For this review, take the finished solid that the model builds, in its own axes (mm). A direction names the side the tool comes from. Give positions to 0.01 mm unless a question says otherwise; leave off trailing zeros. Order: outer loops, then holes, each group sorted by start corner. A loop starts at its lowest first (then second) coordinate and runs counter-clockwise, first axis right, second up. Notation, with made-up numbers: (50, -39.5) -> (72, -39.5) arc R34 ccw to (72, -7.5) -> close; hole circle Ø5 at (20.25, 22.25). An arc over 180 degrees is marked (long way). Return JSON: item names as keys, results as strings. Group by question number.
1) Insertion check: P1, Ø2, axis at y = -1, z = 20.5, coming from the -X side; P2, Ø12.5, axis at x = 149.5, y = 38, coming from the -Z side; P3, Ø1, axis at y = -1, z = -153.5, coming from the +X side. Each pin has a flat end and moves straight along its axis. Give the tip position at first contact, or say it passes through.
2) The part is to be moulded in two halves that separate along Z. For faces 1 (the face through (159, 0, -2)), 2 (the face through (156.7, -1, 159.9)), say which applies: released by +Z, released by -Z, zero draft, split by the parting line, or undercut.
3) Add section C-C (z = 35.5). Give the boundary of the cut face in (x, y).
4) For faces 3 (the face through (159, -2, -2)), 4 (the face through (155.116, 34.439, 1.568)), list the 3-axis set-ups (+Z, -Z, +X, -X, +Y, -Y) from which the entire face can be reached by the end or side of a thin tool; tool diameter is ignored.
5) To check wall thickness, follow line 1 along Z through (x, y) = (160, -0.85); line 2 along X through (y, z) = (-1.5, -160); line 3 along Y through (x, z) = (147, 70). State the ranges of each line that lie inside material, in increasing order.
6) Add section B-B (x = 167). Give the boundary of the cut face in (y, z).
7) Add section A-A (z = 160). Give the boundary of the cut face in (x, y), then the cut area to 3 significant figures.
8) Add section D-D (z = 126). Give the boundary of the cut face in (x, y).
from build123d import *

# Parameters (mm, degrees)
SKIZZE2_W                       = 350
SKIZZE2_H                       = 335
BASIS_BLECH1_DEPTH              = 2
KANTE_LASCHE1_STRIP_CUT_DEPTH   = 224
KANTE_LASCHE1_RELIEF_W          = 14.502816622
KANTE_LASCHE1_RELIEF_H          = 0.3
KANTE_LASCHE1_RELIEF_CUT_DEPTH  = 2
KANTE_LASCHE1_DEPTH             = 224
DURCHGANGSLOCH_F_R_M61_D        = 6.6
DURCHGANGSLOCH_F_R_M61_DEPTH    = 15
DURCHGANGSLOCH_F_R_M61_TIP      = 1.982840043
DURCHGANGSLOCH_F_R_M121_D       = 13.5
SKIZZE30_W                      = 319
SKIZZE30_H                      = 335
SCHNITT_LINEAR_AUSTRAGEN1_DEPTH = 10


# Sheet-metal steps are written as plain solids
with BuildPart() as part:
    # Skizze2 → Basis-Blech1 (new body)
    with BuildSketch(Plane(origin=(0, 0, 0), x_dir=(1, 0, 0), z_dir=(0, 1, 0))):
        Rectangle(SKIZZE2_W, SKIZZE2_H)
    extrude(amount=-BASIS_BLECH1_DEPTH)

    # Kante-Lasche1 strip (across the edge) → Kante-Lasche1 strip cut (cut)
    with BuildSketch(Plane(origin=(175, 0, 112), x_dir=(-0.8660254037844407, -0.49999999999999645, 0), z_dir=(0, 0, -1))):
        Polygon((-11.15, -8.746856578), (1.15, -1.645448267), (0.15, 0.08660254), (-12.15, -7.014805771), align=None)
    extrude(amount=KANTE_LASCHE1_STRIP_CUT_DEPTH, mode=Mode.SUBTRACT)

    # Kante-Lasche1 relief (on the sheet) → Kante-Lasche1 relief cut (cut)
    with BuildSketch(Plane(origin=(174.826794919, 0, 112), x_dir=(-1, 0, 0), z_dir=(0, 1, 0))):
        with Locations((-6.951408311, 0.15)):
            Rectangle(KANTE_LASCHE1_RELIEF_W, KANTE_LASCHE1_RELIEF_H)
        with Locations((-6.951408311, -224.15)):
            Rectangle(KANTE_LASCHE1_RELIEF_W, KANTE_LASCHE1_RELIEF_H)
    extrude(amount=-KANTE_LASCHE1_RELIEF_CUT_DEPTH, mode=Mode.SUBTRACT)

    # Kante-Lasche1 section (across the edge) → Kante-Lasche1 (add)
    with BuildSketch(Plane(origin=(175, 0, 112), x_dir=(-0.8660254037844407, -0.49999999999999645, 0), z_dir=(0, 0, -1))):
        with BuildLine():
            Line((-2, 0.173205081), (-2, 78.267949192))
            Line((-2, 78.267949192), (0, 78.267949192))
            Line((0, 78.267949192), (0, 0.173205081))
            ThreePointArc((0, 0.173205081), (0.05, 0.08660254), (0.15, 0.08660254))
            Line((0.15, 0.08660254), (1.15, -1.645448267))
            ThreePointArc((1.15, -1.645448267), (-0.95, -1.645448267), (-2, 0.173205081))
        make_face()
    extrude(amount=KANTE_LASCHE1_DEPTH)

    # Durchgangsloch für M61
    with Locations(Plane(origin=(0, -2, 0), x_dir=(-1, 0, 0), z_dir=(0, -1, 0))):
        with Locations((-160, -160), (160, -160), (160, 160), (-160, 160)):
            Hole(DURCHGANGSLOCH_F_R_M61_D / 2, depth=DURCHGANGSLOCH_F_R_M61_DEPTH)
            with Locations((0, 0, -(DURCHGANGSLOCH_F_R_M61_DEPTH + DURCHGANGSLOCH_F_R_M61_TIP / 2))):  # 118° drill point
                Cone(0, DURCHGANGSLOCH_F_R_M61_D / 2, DURCHGANGSLOCH_F_R_M61_TIP, mode=Mode.SUBTRACT)

    # Durchgangsloch für M121 (through all)
    with Locations(Plane(origin=(0, 0, 0), x_dir=(1, 0, 0), z_dir=(0, 1, 0))):
        with Locations((-25, 145.5), (-25, -145.5)):
            Hole(DURCHGANGSLOCH_F_R_M121_D / 2)

    # Skizze30 → Schnitt-Linear austragen1 (cut)
    with BuildSketch(Plane.XZ.offset(2)):
        with Locations((-15.5, 0)):
            Rectangle(SKIZZE30_W, SKIZZE30_H)
    extrude(amount=-SCHNITT_LINEAR_AUSTRAGEN1_DEPTH, mode=Mode.SUBTRACT)


solid = part.part
Evaluation:
{
 "1": {"P1": "x = 144", "P2": "z = -112", "P3": "x = 175"},
 "2": {"face 1": "zero draft", "face 2": "undercut"},
 "3": {"outline": "(135.87, 67.78) -> (174.91, 0.15) arc R0.1 cw to (174.83, 0) -> (144, 0) -> (144, -2) -> (174.83, -2) arc R2.1 ccw to (176.65, 1.15) -> (137.6, 68.78) -> close"},
 "4": {"face 3": "+Z, -Z, +X, -X, -Y", "face 4": "+Z, -Z, -X"},
 "5": {"line 1": "-167.5 to -163.3, -156.7 to 156.7, 163.3 to 167.5", "line 2": "144 to 156.7, 163.3 to 175", "line 3": "-2 to 0, 48.5 to 52.5"},
 "6": {"outline": "(-2, -167.5) -> (0, -167.5) -> (0, 167.5) -> (-2, 167.5) -> close; (13.86, -112) -> (17.86, -112) -> (17.86, 112) -> (13.86, 112) -> close"},
 "7": {"outline": "(144, -2) -> (156.7, -2) -> (156.7, 0) -> (144, 0) -> close; (163.3, -2) -> (175, -2) -> (175, 0) -> (163.3, 0) -> close", "area": "48.8 mm^2"},
 "8": {"outline": "(144, -2) -> (175, -2) -> (175, 0) -> (144, 0) -> close"}
}
